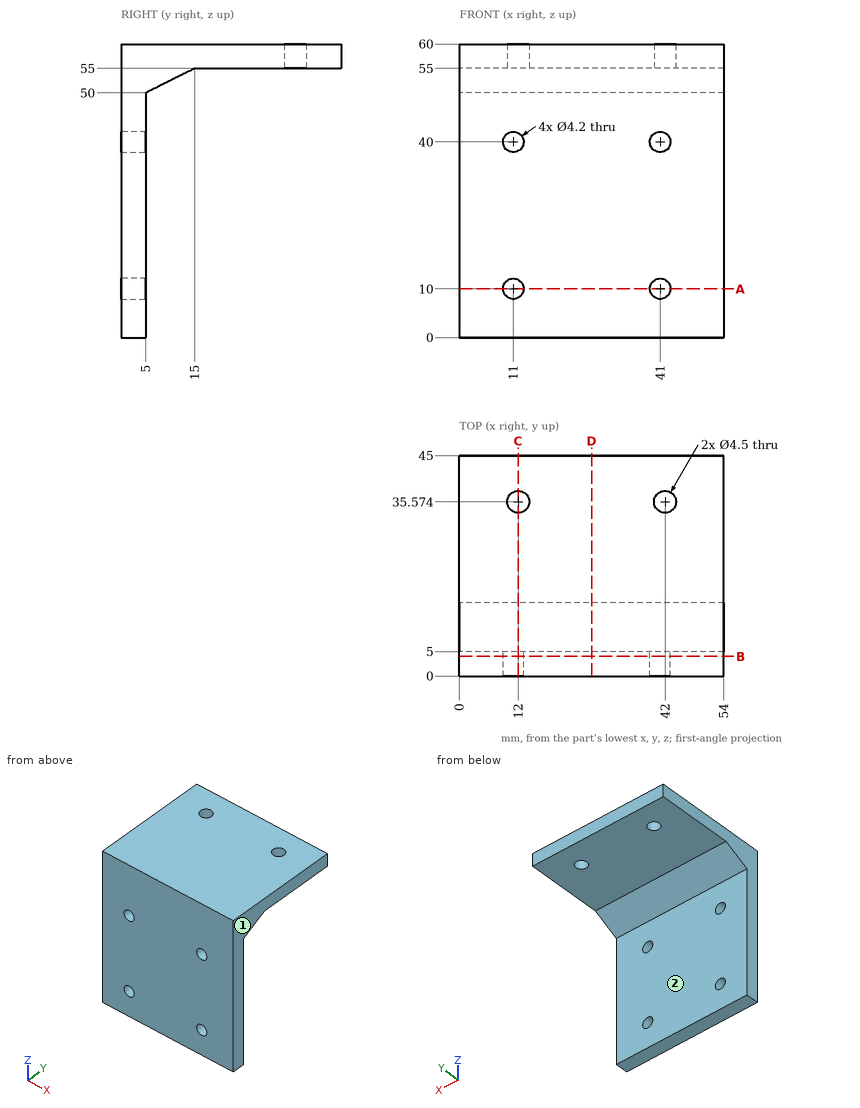
Print and shaded views of the part. All mm, measured from the part's lowest x, y and z. A direction names the side the tool comes from. Give positions to 0.01 mm unless a question says otherwise; leave off trailing zeros. Write each loop counter-clockwise with the first axis right and the second up, starting at its lowest first coordinate (ties: lowest second). Pieces come first, ordered by that corner, then holes. Notation, with made-up numbers: (82.25, -26.5) -> (115.25, -26.5) arc R20 ccw to (115.25, -3.5) -> close; hole circle Ø7 at (75.5, 15). An arc over 180 degrees is marked (long way). Write item = value, one per line.
(1) Slice it at D-D, the plane x = 27. Give the cut face in (y, z), then the cut area to 3 significant figures.
Determined:
outline = (0, 0) -> (5, 0) -> (5, 50) -> (15, 55) -> (45, 55) -> (45, 60) -> (0, 60) -> close
area = 525 mm2
(2) Slice it at A-A, the plane z = 10. Give the cut face in (x, y), then the cut area to 3 significant figures.
Determined:
outline = (0, 0) -> (8.9, 0) -> (8.9, 5) -> (0, 5) -> close; (13.1, 0) -> (38.9, 0) -> (38.9, 5) -> (13.1, 5) -> close; (43.1, 0) -> (54, 0) -> (54, 5) -> (43.1, 5) -> close
area = 228 mm2
(3) Probe line 1 along X through (y, z) = (1.3, 10); line 2 along Y through (x, z) = (43, 5); line 3 along Z through (x, y) = (23, 41). List the from-to ranges inside material, lowest first.
Determined:
line_1 = 0 to 8.9, 13.1 to 38.9, 43.1 to 54
line_2 = 0 to 5
line_3 = 55 to 60
(4) Slice it at B-B, the plane y = 4. Give the cut face in (x, z), then the cut area to 3 significant figures.
Determined:
outline = (0, 0) -> (54, 0) -> (54, 60) -> (0, 60) -> close; hole circle Ø4.2 at (11, 10); hole circle Ø4.2 at (11, 40); hole circle Ø4.2 at (41, 10); hole circle Ø4.2 at (41, 40)
area = 3,180 mm2
(5) Flat gauge pins, fed straight in: P1, Ø6.5, axis at x = 41, z = 40, coming from the +Y side; P2, Ø10, axis at x = 34, y = 12.5, coming from the -Z side; P3, Ø9, axis at x = 40, y = 34.5, coming from the -Z side. Where does each tip first touch, or does it go through?
Determined:
P1 = 5
P2 = 51.25
P3 = 55
(6) Tool access for the marked faces 1 and 2: list every direction of +Z, -Z, +X, -X, +Y, -Y with a clear straight run to the whole face (end or side of a thin tool).
Determined:
face_1 = +Z, -Z, +X, +Y, -Y
face_2 = -Z, +X, -X, +Y
(7) Slice it at C-C, the plane x = 12. Give the cut face in (y, z), then the cut area to 3 significant figures.
Determined:
outline = (0, 0) -> (5, 0) -> (5, 8.15) -> (0, 8.15) -> close; (0, 11.85) -> (5, 11.85) -> (5, 38.15) -> (0, 38.15) -> close; (0, 41.85) -> (5, 41.85) -> (5, 50) -> (15, 55) -> (33.32, 55) -> (33.32, 60) -> (0, 60) -> close; (37.82, 55) -> (45, 55) -> (45, 60) -> (37.82, 60) -> close
area = 466 mm2
